Solid Edge part; units mm, degrees
sketch "Sketch1" plane through (0, 0, 0) normal (1, 0, 0) x (0, 1, 0)
  line L0 (10, -15) -> (-10, -15)
  line L1 (-10, -15) -> (-10, 15)
  line L2 (-10, 15) -> (10, 15)
  line L3 (10, 15) -> (10, -15)
  dimension "D1" = 10
  dimension "D2" = 10
extrude "Protrusion1" add sketch "Sketch1" along normal blind 25
sketch "Sketch2" plane through (25, 0, 0) normal (1, 0, 0) x (0, 1, 0)
  line L0 (10, 15) -> (-8, 15)
  line L1 (-8, 15) -> (-8, -13)
  line L2 (-8, -13) -> (10, -13)
  line L3 (10, -13) -> (10, 15)
extrude "Cutout1" cut sketch "Sketch2" against normal through all
hole "Hole_1" at (20, 5, -13) direction (0, 0, -1) diameter 3.2 end through all
hole "Hole1" at (5, 5, -13) direction (0, 0, -1) diameter 3.2 end through all
hole "Hole_3" at (12.5, -8, 12) direction (0, -1, 0) diameter 2 end through all
hole "Hole2" at (12.5, -8, -4) direction (0, -1, 0) diameter 2 end through all
hole "Hole3" at (20.5, -8, 4) direction (0, -1, 0) diameter 2 end through all
hole "Hole4" at (4.5, -8, 4) direction (0, -1, 0) diameter 2 end through all
hole "Hole_7" at (12.5, -8, 4) direction (0, -1, 0) diameter 9 end through all
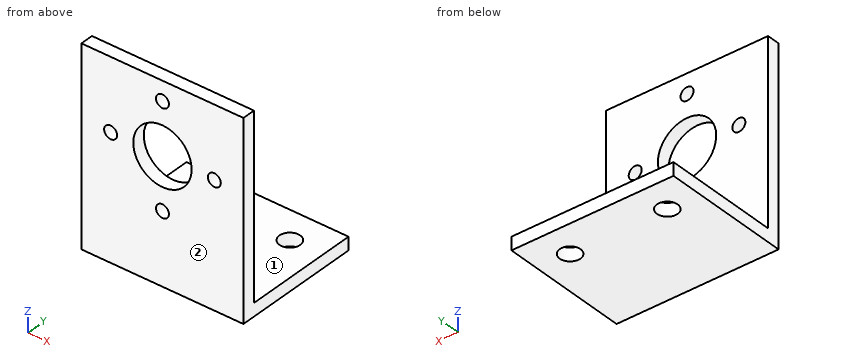
CAD build for the part. Positions are in the model's coordinates, mm. Face numbers are marked on the shaded views. A direction names the side the tool comes from. Round coordinates to 2 decimals unless told otherwise and drop trailing zeros. Write each loop counter-clockwise with the first axis right and the second up, starting at its lowest first coordinate (ties: lowest second). Pieces come first, ordered by that corner, then holes. Notation, with made-up numbers: M 50.5,-35.75 L 95.5,-35.75 A27 cw 95.5,-17.75 Z; hole C 32.5,-26 d2. An arc over 180 degrees is marked long. One line per question, with ' | ' between items.
1. Cut at D-D on z = 12. Write the cut outline in (x, y).
Working result:
outline: M 0,-10 L 11.5,-10 L 11.5,-8 L 0,-8 Z; M 13.5,-10 L 25,-10 L 25,-8 L 13.5,-8 Z
2. Which spindle directions (+Z, -Z, +X, -X, +Y, -Y) get a long thin tool onto all of the face, cutting with end or side? Do the marked faces 1 and 2. Say none if no direction does.
Working result:
face 1: +Z, +X, -X, +Y | face 2: +Z, -Z, +X, -X, -Y
3. Cut at C-C on x = 20. Write the cut outline in (y, z), and give its area (3 significant figures).
Working result:
outline: M -10,-15 L 3.4,-15 L 3.4,-13 L -8,-13 L -8,3.13 L -10,3.13 Z; M -10,4.87 L -8,4.87 L -8,15 L -10,15 Z; M 6.6,-15 L 10,-15 L 10,-13 L 6.6,-13 Z | area: 86.1 mm2
4. Probe L1, parallel to X at y = 5, z = -14.05; L2, parallel to Z at x = 12.5, y = -9.2; L3, parallel to Z at x = 20.5, y = -9.5. List the from-to ranges inside material, lowest first. Write a range as from..to.
Working result:
L1: 0..3.4, 6.6..18.4, 21.6..25 | L2: -15..-5, -3..-0.5, 8.5..11, 13..15 | L3: -15..3, 5..15
5. Cut at B-B on z = 4. Write the cut outline in (x, y).
Working result:
outline: M 0,-10 L 3.5,-10 L 3.5,-8 L 0,-8 Z; M 5.5,-10 L 8,-10 L 8,-8 L 5.5,-8 Z; M 17,-10 L 19.5,-10 L 19.5,-8 L 17,-8 Z; M 21.5,-10 L 25,-10 L 25,-8 L 21.5,-8 Z
6. Pin check, flat tips, straight feed: pin 1 Ø4 at (x, z) = (14.5, -7.5) entering from +Y; pin 2 Ø1.5 at (x, y) = (12.5, -4.5) entering from +Z. Stop position of each tip, or through.
Working result:
pin 1: y = -8 | pin 2: z = -13
7. Cut at A-A on y = 5. Write the cut outline in (x, z), and give its area (3 significant figures).
Working result:
outline: M 0,-15 L 3.4,-15 L 3.4,-13 L 0,-13 Z; M 6.6,-15 L 18.4,-15 L 18.4,-13 L 6.6,-13 Z; M 21.6,-15 L 25,-15 L 25,-13 L 21.6,-13 Z | area: 37.2 mm2
